Geometry check sheet. Reference: the model listing, model coordinates, mm. Face numbers are marked on the shaded views. A direction names the side the tool comes from. Give positions to 0.01 mm unless a question says otherwise; leave off trailing zeros. Write each loop counter-clockwise with the first axis right and the second up, starting at its lowest first coordinate (ties: lowest second). Pieces come first, ordered by that corner, then holes. Notation, with made-up numbers: M 53.25,32 L 77.25,32 A37 cw 77.25,68 Z; hole C 25.5,34 d1. An arc over 180 degrees is marked long. One line per item, written item: value. Start each with the question number.
1. Release check for a two-part mould opening along X. For the marked faces 3, 4, 5 and 6 record: pulls with the +X half, pulls with the -X half, needs draft (parallel to the pull), parting line crosses it, or undercut.
2. Tool access check on the marked faces 1 and 2. Record the directions out of +Z, -Z, +X, -X, +Y, -Y that give a thin tool (end or side, any length) a straight path to the whole face; none if there is none.
3. Cross-section at C-C on z = 8.75. Count the separate pieces of the cut face and the enclosed holes in it, then the cut area to 3 significant figures.
4. Scan lines: line 1 (Y direction, x = 0, z = 8.35); line 2 (Y direction, x = 0, z = 2.65); line 3 (X direction, y = 19.05, z = 1.4). Record each from-to range of solid material in increasing order.
5. Gauge pin test, flat end, axial feed: pin 1 (3 mm diameter, centred on x = 2, y = -15, fed in from -Z). Record the tip position at first contact, or that the pin passes through.
6. Cross-section at A-A on x = 0. Record the cut outline in (y, z) (1 decimal).
7. Cross-section at B-B on y = 19.05. Record the cut outline in (x, z) (1 decimal), then the cut area to 3 significant figures.
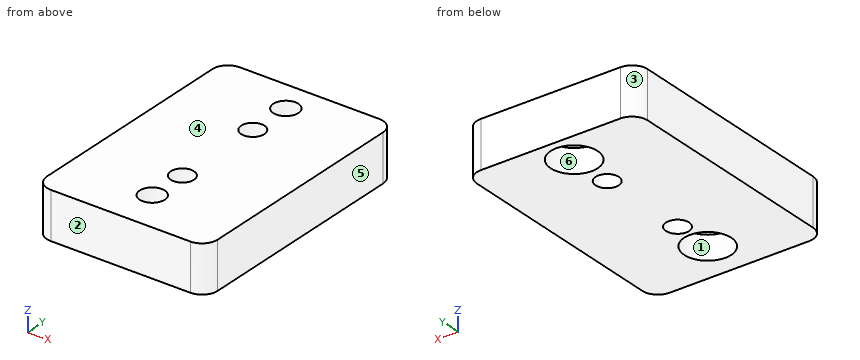
Autodesk Inventor part; units mm, degrees
ref_plane "YZ Plane" through (0, 0, 0) normal (1, 0, 0) x (0, 1, 0)
ref_plane "XZ Plane" through (0, 0, 0) normal (0, 1, 0) x (-1, 0, 0)
ref_plane "XY Plane" through (0, 0, 0) normal (0, 0, 1) x (1, 0, 0)
sketch "Sketch1" plane through (0, 0, 0) normal (0, 0, 1) x (1, 0, 0)
  line L0 (-17.3375, 25.4) -> (17.3375, 25.4)
  line L1 (17.3375, 25.4) -> (17.3375, -25.4)
  line L2 (17.3375, -25.4) -> (-17.3375, -25.4)
  line L3 (-17.3375, -25.4) -> (-17.3375, 25.4)
  line L4 (-17.3375, 25.4) -> (17.3375, -25.4) construction
  line L5 (17.3375, 25.4) -> (-17.3375, -25.4) construction
  line L6 (0, 19.05) -> (0, -16.871) construction
  line L7 (0, 10.16) -> (0, -8.756) construction
  point P0 (0, 0)
  point P1 (0, 0.702)
  point P2 (0, 25.4)
  point P3 (0, 1.0895)
  dimension "d0" = 34.675
  dimension "d1" = 50.8
  dimension "d3" = 18.916
  dimension "d4" = 15.24
  dimension "d23" = 35.921
  dimension "d26" = 6.35
extrude "Extrusion1" add sketch "Sketch1" along normal blind 9.525
hole "Hole1" at (0, 19.05, 0) at (0, -16.871, 0) direction (0, 0, 1) diameter 5.1054 end through all counterbore diameter 9.525 counterbore depth 4.826
hole "Hole2" at (0, -8.756, 0) at (0, 10.16, 0) direction (0, 0, 1) diameter 4.7 end through all
fillet "Fillet1" radius 3.175 4 edges at (17.3375, 25.4, 4.7625) (-17.3375, 25.4, 4.7625) (-17.3375, -25.4, 4.7625) (17.3375, -25.4, 4.7625)
properties part number "anderson battery connectorAnderson adapter" material "ABS Plastic"
Report:
1. face 3: pulls with the -X half
1. face 4: needs draft
1. face 5: pulls with the +X half
1. face 6: undercut
2. face 1: -Z
2. face 2: +Z, -Z, +X, -X, -Y
3. separate pieces: 1
3. enclosed holes: 4
3. area: 1,680 mm^2
4. line 1: y = -25.4 to -19.42, -14.32 to -11.11, -6.41 to 7.81, 12.51 to 16.5, 21.6 to 25.4
4. line 2: y = -25.4 to -21.63, -12.11 to -11.11, -6.41 to 7.81, 12.51 to 14.29, 23.81 to 25.4
4. line 3: x = -17.34 to -4.76, 4.76 to 17.34
5. pin 1: stops at z = 4.83
6. outline: M -25.4,0 L -21.6,0 L -21.6,4.8 L -19.4,4.8 L -19.4,9.5 L -25.4,9.5 Z; M -14.3,4.8 L -12.1,4.8 L -12.1,0 L -11.1,0 L -11.1,9.5 L -14.3,9.5 Z; M -6.4,0 L 7.8,0 L 7.8,9.5 L -6.4,9.5 Z; M 12.5,0 L 14.3,0 L 14.3,4.8 L 16.5,4.8 L 16.5,9.5 L 12.5,9.5 Z; M 21.6,4.8 L 23.8,4.8 L 23.8,0 L 25.4,0 L 25.4,9.5 L 21.6,9.5 Z
7. outline: M -17.3,0 L -4.8,0 L -4.8,4.8 L -2.6,4.8 L -2.6,9.5 L -17.3,9.5 Z; M 2.6,4.8 L 4.8,4.8 L 4.8,0 L 17.3,0 L 17.3,9.5 L 2.6,9.5 Z
7. area: 260 mm^2
